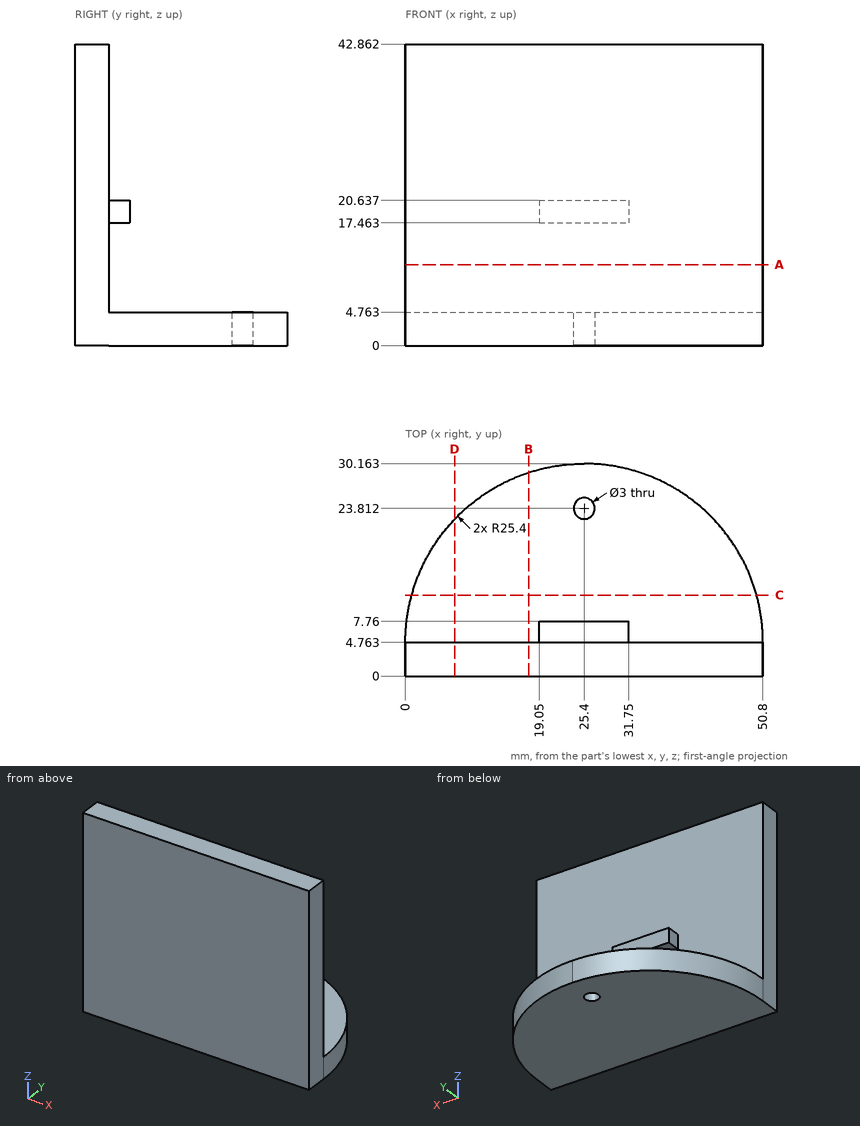
Answer from the drawing. Dimensions are ordinates in mm from the lowest x, y and z of the part. Coordinates: 2 decimals unless noted, no trailing zeros. Loops run counter-clockwise (first coordinate to the right, second up) from the corner with the lowest first, then second, coordinate; pieces in that order, holes last.
1) Section B-B (x = 17.5) is taken. Give the vertices of the cut face in (y, z).
Results:
outline: (0, 0) - (28.9, 0) - (28.9, 4.76) - (4.76, 4.76) - (4.76, 42.86) - (0, 42.86) - close
2) Flat-ended cylindrical pins translate along their axes: pin 1 (12.5 mm diameter, centred on x = 28, y = 12.5, fed in from +Z); pin 2 (4 mm diameter, centred on x = 19, y = 18, fed in from +Z); pin 3 (8 mm diameter, centred on x = 38, z = 14, fed in from +Y). Find the tip coordinate at first contact, or state that the pin passes through.
Results:
pin 1: stops at z = 20.64
pin 2: stops at z = 4.76
pin 3: stops at y = 4.76
3) Section A-A (z = 11.5) is taken. Give the vertices of the cut face in (x, y), plus the area to 3 significant figures.
Results:
outline: (0, 0) - (50.8, 0) - (50.8, 4.76) - (0, 4.76) - close
area: 242 mm2
4) Section D-D (x = 7) is taken. Give the vertices of the cut face in (y, z).
Results:
outline: (0, 0) - (22.27, 0) - (22.27, 4.76) - (4.76, 4.76) - (4.76, 42.86) - (0, 42.86) - close
5) Section C-C (y = 11.5) is taken. Give the vertices of the cut face in (x, z), plus the area to 3 significant figures.
Results:
outline: (0.91, 0) - (49.89, 0) - (49.89, 4.76) - (0.91, 4.76) - close
area: 233 mm2
6) Consider probe 1 along Y at (x, z) = (25.4, 1.2); probe 2 along Z at (x, y) = (43, 22.5). Determine where each line is inside the solid, lowest interval first.
Results:
probe 1: y = 0 to 22.31, 25.31 to 30.16
probe 2: z = 0 to 4.76
